```python
from build123d import *

# Parameters (mm, degrees)
SKETCH_W        = 45
SKETCH_H        = 70
SKETCH_R        = 2.25
PAD_DEPTH       = 15
SKETCH001_R     = 7.6
POCKET_DEPTH    = 70.001
SKETCH002_R     = 4.6
POCKET001_DEPTH = 4


with BuildPart() as part:
    # Sketch → Pad (new body)
    with BuildSketch(Plane.XY):
        Rectangle(SKETCH_W, SKETCH_H)
        with Locations((-16.7, 30)):
            Circle(SKETCH_R, mode=Mode.SUBTRACT)
        with Locations((16.7, 30)):
            Circle(SKETCH_R, mode=Mode.SUBTRACT)
        with Locations((-16.7, -30)):
            Circle(SKETCH_R, mode=Mode.SUBTRACT)
        with Locations((16.7, -30)):
            Circle(SKETCH_R, mode=Mode.SUBTRACT)
        with Locations((-16.7, 0)):
            Circle(SKETCH_R, mode=Mode.SUBTRACT)
        with Locations((16.7, 0)):
            Circle(SKETCH_R, mode=Mode.SUBTRACT)
        with Locations((16.7, 15)):
            Circle(SKETCH_R, mode=Mode.SUBTRACT)
        with Locations((-16.7, 15)):
            Circle(SKETCH_R, mode=Mode.SUBTRACT)
    extrude(amount=PAD_DEPTH)

    # Sketch001 → Pocket (cut, through all)
    with BuildSketch(Plane.XZ.offset(35)):
        with Locations((0, 15)):
            Circle(SKETCH001_R)
    extrude(amount=-POCKET_DEPTH, mode=Mode.SUBTRACT)

    # Sketch002 → Pocket001 (cut)
    with BuildSketch(Plane.XY.offset(15)):
        with Locations((-16.7, 15)):
            Circle(SKETCH002_R)
        with Locations((16.7, 15)):
            Circle(SKETCH002_R)
    extrude(amount=-POCKET001_DEPTH, mode=Mode.SUBTRACT)


solid = part.part
```
Source: CAD feature listing. Evaluate the final solid. Frame: model axes, mm. A direction names the side the tool comes from. Round coordinates to 2 decimals unless told otherwise and drop trailing zeros. Loops run counter-clockwise (first coordinate to the right, second up) from the corner with the lowest first, then second, coordinate; pieces in that order, holes last. Notation, with made-up numbers: M -12,11.25 L 3,11.25 A22 ccw 3,37.25 Z; hole C 47,-29.5 d2. An arc over 180 degrees is marked long. Use a Markdown table: item, result. Add a question column.
1. Cut plane B-B, the plane y = 15. Output: boundary loops of the cut face in (x, z), and give its area (3 significant figures).
2. Pull-direction query (X, two-part tool) for faces 1 (the flat face through (22.5, 0, 7)), 2 (the cylindrical face through (-18.486, 13.631, 5.423)), 3 (the flat face through (0, 35, 7)); classes: +X half, -X half, draft (parallel to the pull), parting line (faces both ways), or undercut.
3. Cut plane C-C, the plane z = 5.75. State how many separate pieces and enclosed holes the cut face has, and give its area (3 significant figures).
4. Contact query for flat-ended pins moving along their axis: pin 1 (4 mm diameter, centred on x = 16.7, y = 0, fed in from -Z); pin 2 (4.5 mm diameter, centred on x = 15.5, y = 14, fed in from +Z). Output: stop coordinate, or through.
5. Cut plane A-A, the plane x = -16.7. Output: boundary loops of the cut face in (y, z), and give its area (3 significant figures).
6. Ray query, line 1 along Y through (x, z) = (16.7, 13.2); line 2 along Y through (x, z) = (-16.7, 4.25); line 3 along X through (y, z) = (1.5, 7). Return the intervals inside material, ascending. Write a range as [from, to].
7. Cut plane D-D, the plane y = -30. Output: boundary loops of the cut face in (x, z), and give its area (3 significant figures).
8. Set-up query: faces 4 (the cylindrical face through (-18.486, -31.369, 7.395)), 5 (the cylindrical face through (21.09, 16.38, 13.03)). Return all of +Z, -Z, +X, -X, +Y, -Y with unobstructed straight access to the full face (end or side cutting, diameter ignored); none if empty.
Solution:
| question | item | result |
|---|---|---|
| 1 | outline | M -22.5,0 L -18.95,0 L -18.95,11 L -21.3,11 L -21.3,15 L -22.5,15 Z; M -14.45,0 L 14.45,0 L 14.45,11 L 12.1,11 L 12.1,15 L 7.6,15 A7.6 cw -7.6,15 L -12.1,15 L -12.1,11 L -14.45,11 Z; M 18.95,0 L 22.5,0 L 22.5,15 L 21.3,15 L 21.3,11 L 18.95,11 Z |
| 1 | area | 412 mm2 |
| 2 | face 1 | +X half |
| 2 | face 2 | undercut |
| 2 | face 3 | draft |
| 3 | separate pieces | 1 |
| 3 | enclosed holes | 8 |
| 3 | area | 3,020 mm2 |
| 4 | pin 1 | passes through |
| 4 | pin 2 | stops at z = 11 |
| 5 | outline | M -35,0 L -32.25,0 L -32.25,15 L -35,15 Z; M -27.75,0 L -2.25,0 L -2.25,15 L -27.75,15 Z; M 2.25,0 L 12.75,0 L 12.75,11 L 10.4,11 L 10.4,15 L 2.25,15 Z; M 17.25,0 L 27.75,0 L 27.75,15 L 19.6,15 L 19.6,11 L 17.25,11 Z; M 32.25,0 L 35,0 L 35,15 L 32.25,15 Z |
| 5 | area | 761 mm2 |
| 6 | line 1 | y = [-35, -32.25], [-27.75, -2.25], [2.25, 10.4], [19.6, 27.75], [32.25, 35] |
| 6 | line 2 | y = [-35, -32.25], [-27.75, -2.25], [2.25, 12.75], [17.25, 27.75], [32.25, 35] |
| 6 | line 3 | x = [-22.5, -18.38], [-15.02, 15.02], [18.38, 22.5] |
| 7 | outline | M -22.5,0 L -18.95,0 L -18.95,15 L -22.5,15 Z; M -14.45,0 L 14.45,0 L 14.45,15 L 7.6,15 A7.6 cw -7.6,15 L -14.45,15 Z; M 18.95,0 L 22.5,0 L 22.5,15 L 18.95,15 Z |
| 7 | area | 449 mm2 |
| 8 | face 4 | +Z, -Z |
| 8 | face 5 | +Z |
